Can you work these out from the drawing? Everything is in mm from the part's minimum corner. Coordinates: 2 decimals unless noted, no trailing zeros. Write each loop counter-clockwise with the first axis right and the second up, starting at its lowest first coordinate (ties: lowest second). Pieces come first, ordered by that corner, then holes.
(1) For pin 1 Ø6 at (x, z) = (79, 13) entering from +Y, with a flat end and sliding along its axis, tell me the tip position at first contact or that it passes through.
(2) Imagine slicing it at B-B, the plane x = 81.5. List the corners of the cut face in (y, z) for me, plus the area to 3 significant figures.
(3) Please list where these lines run through material, in increasing order: probe 1 along Y at (x, z) = (34.5, 2.75); probe 2 along Y at (x, z) = (50, 5); probe 3 along X at (y, z) = (527, 17).
(4) Imagine slicing it at A-A, the plane z = 12.5. List the corners of the cut face in (x, y) for me (3 decimals).
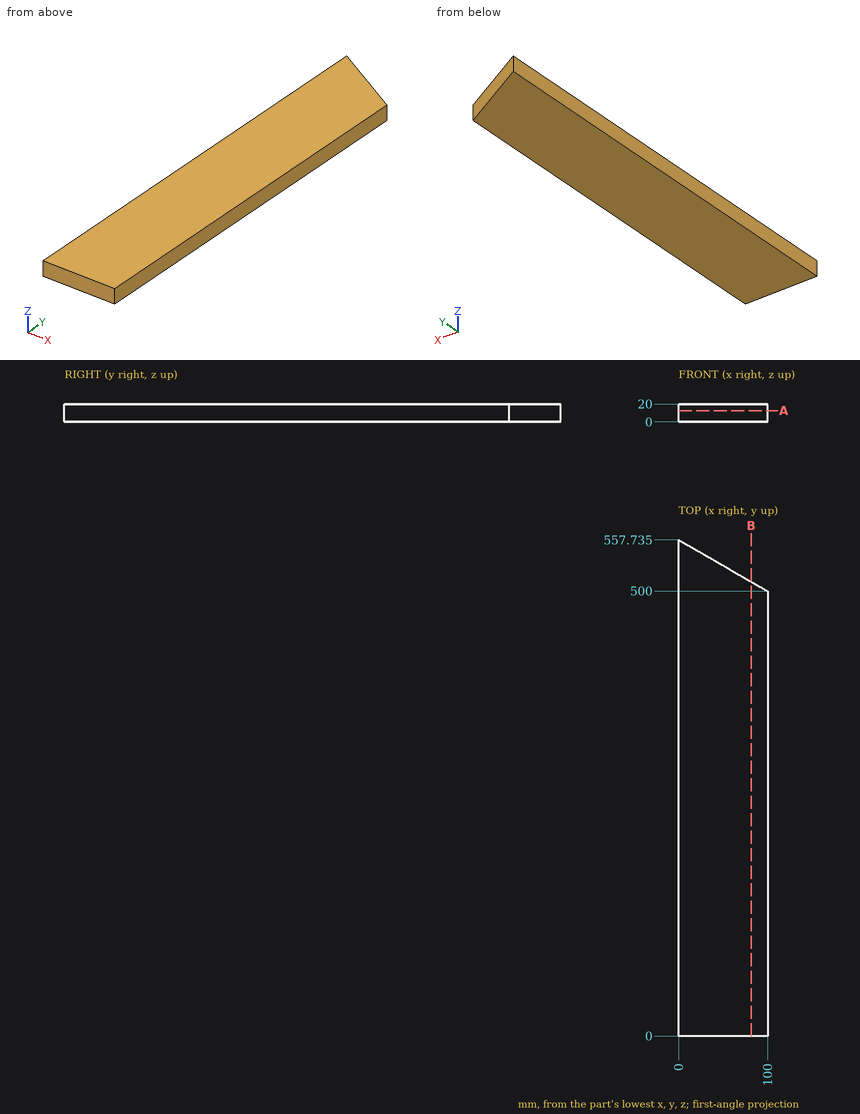
Recorded:
1. pin 1: stops at y = 513.86
2. outline: (0, 0) - (510.68, 0) - (510.68, 20) - (0, 20) - close
2. area: 10,200 mm2
3. probe 1: y = 0 to 537.82
3. probe 2: y = 0 to 528.87
3. probe 3: x = 0 to 53.23
4. outline: (0, 0) - (100, 0) - (100, 500) - (0, 557.735) - close
